CAD build for the part. Positions are in the model's coordinates, mm. A direction names the side the tool comes from. Coordinates: 2 decimals unless noted, no trailing zeros. Loops run counter-clockwise (first coordinate to the right, second up) from the corner with the lowest first, then second, coordinate; pieces in that order, holes last. Notation, with made-up numbers: M -1.75,59.5 L 53.25,59.5 A22 cw 53.25,72.5 Z; hole C 17,26 d11. An arc over 180 degrees is marked long. Answer as a JSON object with one key per item and string values. Group by question number.
Autodesk Inventor part; units mm, degrees
ref_plane "YZ Plane" through (0, 0, 0) normal (1, 0, 0) x (0, 1, 0)
ref_plane "XZ Plane" through (0, 0, 0) normal (0, 1, 0) x (-1, 0, 0)
ref_plane "XY Plane" through (0, 0, 0) normal (0, 0, 1) x (1, 0, 0)
sketch "Sketch1" plane through (0, 0, 0) normal (0, 1, 0) x (-1, 0, 0)
  point P0 (0, 0)
sketch "Sketch2" plane through (0, 0, 0) normal (0, 1, 0) x (-1, 0, 0)
  line L0 (0, 0) -> (0, -50)
  line L1 (0, -50) -> (-25, -50)
  line L2 (-40, -35) -> (-40, -15)
  line L3 (-25, 0) -> (0, 0)
  line L4 (-25, -50) -> (-40, -35)
  line L5 (-25, 0) -> (-40, -15)
  line L6 (-9, -35) -> (-9, -41.5)
  line L7 (-9, -41.5) -> (-21, -41.5)
  line L8 (-21, -41.5) -> (-21, -19)
  line L9 (-21, -19) -> (-9, -19)
  line L10 (-9, -19) -> (-9, -35)
  circle A0 centre (-15, -15) radius 3
  line L11 (0, -25) -> (-40, -25)
  circle A1 centre (-15, -15) radius 1.5
  line L12 (0, 0) -> (5, 0)
  line L13 (5, 0) -> (5, -50)
  line L14 (5, -50) -> (0, -50)
  circle A2 centre (-36, -21) radius 3
  circle A3 centre (-36, -29) radius 3
  circle A4 centre (-36, -21) radius 1.5
  circle A5 centre (-36, -29) radius 1.5
  dimension "d0" = 50
  dimension "d1" = 25
  dimension "d4" = 20
  dimension "d7" = 6.5
  dimension "d8" = 12
  dimension "d9" = 22.5
  dimension "d10" = 6
  dimension "d13" = 3
  dimension "d16" = 5
  dimension "d17" = 6
  dimension "d18" = 6
  dimension "d19" = 3
  dimension "d20" = 3
extrude "Extrusion1" add sketch "Sketch2" along normal blind 8 contours A0 | A2 | A3
extrude "Extrusion2" add sketch "Sketch2" along normal blind 4 contours L0 L11 L10 L9 L8 L2 L5 L3 | L0 L1 L4 L2 L11 L8 L7 L6 L10
extrude "Extrusion3" add sketch "Sketch2" along normal blind 31.807 contours L12 L13 L14 L0
sketch "Szkic4" plane through (-5, 0, -50) normal (-1, 0, 0) x (0, 0, 1)
  line L0 (0, 0) -> (50, 0)
  line L1 (50, 0) -> (50, 31.807)
  line L2 (0, 31.807) -> (50, 31.807)
  line L3 (0, 0) -> (0, 31.807)
  line L4 (38, 21.6151) -> (12, 21.6151)
  line L5 (25, 21.6151) -> (25, 0)
  line L6 (25, 21.6151) -> (25, 31.807)
  line L7 (12, 21.6151) -> (12, 31.807)
  line L8 (12, 21.6151) -> (12, 0)
  dimension "d32" = 31.807
  dimension "d33" = 50
  dimension "d34" = 26
  dimension "d35" = 12
  dimension "d36" = 12
  dimension "d37" = 13
extrude "Wyciągnięcie proste5" add sketch "Szkic4" along normal blind 30 contours L8 L4 L5 L0 | L7 L2 L6 L4
sketch "Szkic5" plane through (-5, 0, -38) normal (0, 0, -1) x (-1, 0, 0)
  line L0 (0, 0) -> (30, 0)
  line L1 (0, 31.807) -> (30, 31.807)
  line L2 (30, 31.807) -> (30, 0)
  line L3 (0, 0) -> (0, 31.807)
  line L4 (0, 0) -> (30, 0)
  line L5 (30, 31.807) -> (30, 0)
  line L6 (0, 31.807) -> (30, 31.807)
  point P0 (-5, 0)
  point P1 (22, 8)
  point P2 (22, 23.807)
  point P3 (8, 8)
  point P4 (8, 23.807)
  dimension "d40" = 8
  dimension "d41" = 8
  dimension "d42" = 8
  dimension "d43" = 8
  dimension "d51" = 8
  dimension "d52" = 8
  dimension "d53" = 8
  dimension "d54" = 8
hole "Otwór1" at (-27, 8, -38) at (-27, 23.807, -38) at (-13, 8, -38) at (-13, 23.807, -38) direction (0, 0, 1) diameter 3.242 end through all
sketch "Szkic6" plane through (-5, 0, -38) normal (0, 0, -1) x (-1, 0, 0)
  circle A0 centre (8, 23.807) radius 1.621
  circle A1 centre (8, 8) radius 1.621
  circle A2 centre (22, 23.807) radius 1.621
  circle A3 centre (22, 8) radius 1.621
  line L0 (0, 0) -> (0, 31.807)
  line L1 (0, 0) -> (30, 0)
  line L2 (30, 31.807) -> (30, 0)
  line L3 (0, 31.807) -> (30, 31.807)
  circle A4 centre (8, 23.807) radius 4
  circle A5 centre (22, 23.807) radius 4
  circle A6 centre (22, 8) radius 4
  circle A7 centre (8, 8) radius 4
  point P0 (-5, 0)
  dimension "d55" = 8
  dimension "d56" = 8
  dimension "d57" = 8
  dimension "d58" = 8
extrude "Wyciągnięcie proste6" cut sketch "Szkic6" against normal blind 9 contours A4 | A5 | A6 | A7
properties part number "podstawachwytak"
Item 1: Pin check, flat tips, straight feed: pin 1 (4 mm diameter, centred on x = -13, y = 23.807, fed in from +Z); pin 2 (1.5 mm diameter, centred on y = 16.5, z = -18.5, fed in from -X); pin 3 (5 mm diameter, centred on x = -13, y = 23.807, fed in from -Z); pin 4 (1.8 mm diameter, centred on x = 36.5, z = -21, fed in from +Y). Stop position of each tip, or through.
Item 2: Drill centre lines: L1, parallel to Z at x = 36, y = 5.5; L2, parallel to Y at x = -27, z = -27.2; L3, parallel to Z at x = 15, y = 2. Where is each one in solid material? Low to high. Write a range as from..to.
Item 3: Pull direction Z, two halves, no side cores. Call faces 1 (the flat face through (-20, 16, -38)), 2 (the cylindrical face through (-10.05, 26.51, -33.56)), 3 (the flat face through (15, 2, -19)), 4 (the cylindrical face through (16.5, 3.94, -15.07)): released by +Z, released by -Z, zero draft, split by the parting line, or undercut.
Item 4: Slice it at D-D, the plane x = 10. Write the cut outline in (y, z), then the cut area to 3 significant figures.
Item 5: Slice it at C-C, the plane z = -37. Write the cut outline in (x, y).
Item 6: Slice it at B-B, the plane z = -21. Write the cut outline in (x, y).
Item 7: Slice it at A-A, the plane x = -13. Write the cut outline in (y, z), then the cut area to 3 significant figures.
Item 8: Tool access for faces 5 (the cylindrical face through (-23.8, 5.6, -33.6)), 6 (the flat face through (13.7, 8, -16.3)), 7 (the cylindrical face through (39, 6, -21)): list every direction of +Z, -Z, +X, -X, +Y, -Y with a clear straight run to the whole face (end or side of a thin tool).
Computed:
{
 "1": {"pin 1": "z = -25", "pin 2": "x = -5", "pin 3": "z = -29", "pin 4": "through"},
 "2": {"L1": "-32..-30.5, -27.5..-26, -24..-22.5, -19.5..-18", "L2": "0..6.38, 9.62..22.19, 25.43..31.81", "L3": "-50..-41.5, -19..-16.5, -13.5..0"},
 "3": {"face 1": "released by -Z", "face 2": "zero draft", "face 3": "undercut", "face 4": "undercut"},
 "4": {"outline": "M 0,-50 L 4,-50 L 4,-41.5 L 0,-41.5 Z; M 0,-19 L 4,-19 L 4,0 L 0,0 Z", "area": "110 mm2"},
 "5": {"outline": "M -35,0 L 9,0 L 9,4 L 0,4 L 0,31.81 L -35,31.81 Z; M 21,0 L 38,0 L 38,4 L 21,4 Z; hole C -27,8 d8; hole C -27,23.81 d8; hole C -13,8 d8; hole C -13,23.81 d8"},
 "6": {"outline": "M -5,0 L 9,0 L 9,4 L 0,4 L 0,31.81 L -5,31.81 Z; M 21,0 L 34.5,0 L 34.5,8 L 33,8 L 33,4 L 21,4 Z; M 37.5,0 L 40,0 L 40,4 L 39,4 L 39,8 L 37.5,8 Z"},
 "7": {"outline": "M 0,-38 L 4,-38 L 4,-29 L 6.38,-29 L 6.38,-25 L 0,-25 Z; M 9.62,-29 L 12,-29 L 12,-38 L 19.81,-38 L 19.81,-29 L 22.19,-29 L 22.19,-25 L 9.62,-25 Z; M 25.43,-29 L 27.81,-29 L 27.81,-38 L 31.81,-38 L 31.81,-25 L 25.43,-25 Z", "area": "244 mm2"},
 "8": {"face 5": "-Z", "face 6": "+Z, -Z, +X, +Y", "face 7": "+Y"}
}
